Verification items for this drawing (mm, ordinates from the low corner). Give positions to 0.01 mm unless a question says otherwise; leave off trailing zeros. Write each loop counter-clockwise with the first axis right and the second up, starting at its lowest first coordinate (ties: lowest second). Pieces come first, ordered by that corner, then holes. Notation, with made-up numbers: (-2, 55.5) -> (40, 55.5) arc R34 ccw to (40, 92.5) -> close; hole circle Ø10 at (19, 72.25). An arc over 180 degrees is marked (long way). One line per item, written item: value.
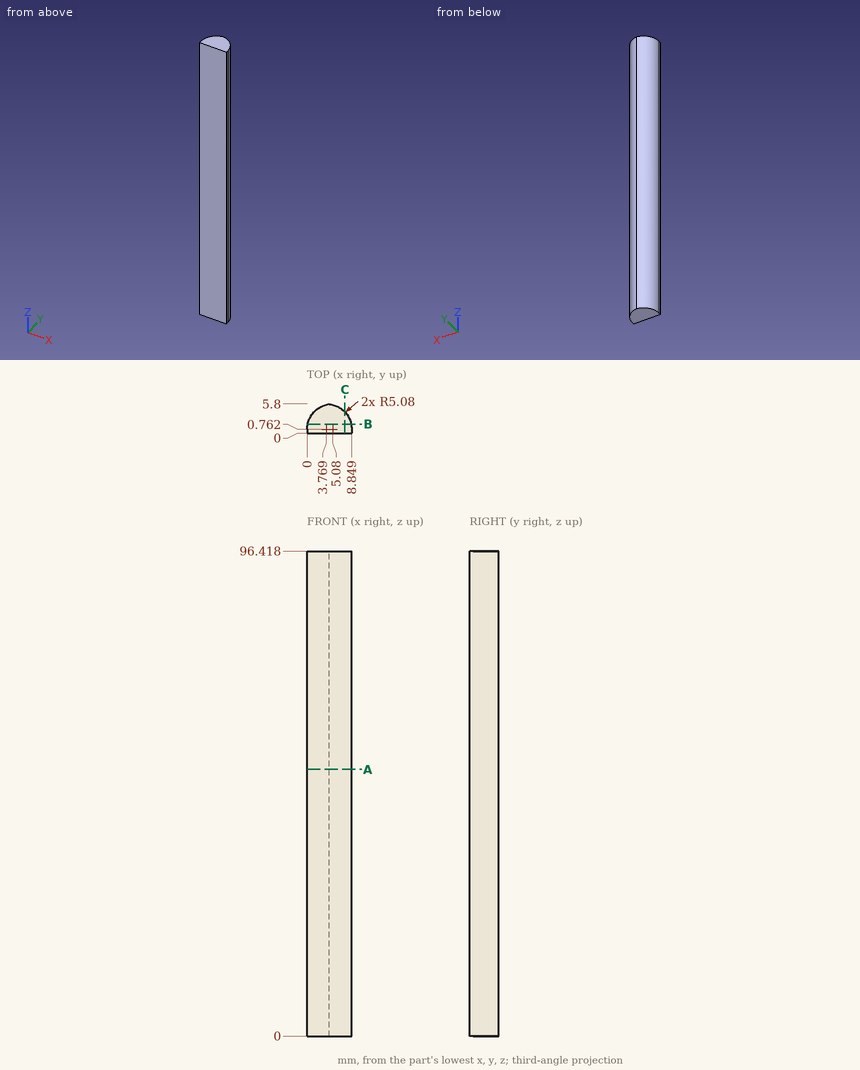
1) Sectioned sample at A-A on z = 53. Record the cut outline in (x, y) (1 decimal).
Verdict:
outline: (0, 0) -> (8.8, 0) -> (8.8, 0.8) arc R5.1 ccw to (4.4, 5.8) arc R5.1 ccw to (0, 0.8) -> close
2) Scan lines: probe 1 along Y at (x, z) = (4.5, 14); probe 2 along X at (y, z) = (2.2, 67); probe 3 along Y at (x, z) = (2.25, 82.5). Record each from-to range of solid material in increasing order.
Verdict:
probe 1: 0 to 5.79
probe 2: 0.21 to 8.64
probe 3: 0 to 4.98
3) Sectioned sample at B-B on y = 1.8. Record the cut outline in (x, z).
Verdict:
outline: (0.11, 0) -> (8.74, 0) -> (8.74, 96.42) -> (0.11, 96.42) -> close
4) Sectioned sample at C-C on x = 7.5. Record the cut outline in (y, z), plus the area to 3 significant figures.
Verdict:
outline: (0, 0) -> (4.21, 0) -> (4.21, 96.42) -> (0, 96.42) -> close
area: 406 mm^2
5) Depth check by flat-ended pin: pin 1 Ø5 at (x, z) = (1, 72.5) entering from +Y; pin 2 Ø2 at (y, z) = (4.5, 17) entering from +X. Enter the tip coordinate at first touch or a pass-through.
Verdict:
pin 1: y = 5.59
pin 2: x = 8.05
